Here's how the part is built. I have some questions about the finished solid (model axes, mm). A direction names the side the tool comes from. Give positions to 0.01 mm unless a question says otherwise; leave off trailing zeros. Order: outer loops, then holes, each group sorted by start corner. A loop starts at its lowest first (then second) coordinate and runs counter-clockwise, first axis right, second up. Notation, with made-up numbers: (15.25, 20) -> (55.25, 20) arc R29 ccw to (55.25, 57) -> close; hole circle Ø2 at (17.25, 64). An arc over 180 degrees is marked (long way). Write each question's results on one line, items separated by ' | '. Start each with the question number.
Q1. For faces 4 (the face through (-24, 17, -21)), 5 (the face through (1.92, 5.03, 21.45)), 6 (the face through (14.33, 16.79, -36.84)), 7 (the face through (20.49, 16.79, -36.75)), 8 (the face through (-14.328, 16.79, -6.367)), which set-ups out of +Z, -Z, +X, -X, +Y, -Y let a thin tool reach every point of the face, with its end or its side?
Q2. Thinking about a two-plate mould opening in X: for faces 1 (the face through (-19.01, 16.79, -8.22)), 2 (the face through (-13.88, 0.99, 24.24)), 3 (the face through (27.5, 1, -23)), which applies, pulls with the +X half, pulls with the -X half, needs draft (parallel to the pull), parting line crosses it, or undercut?
Q3. Imagine slicing it at B-B, the plane z = -21. Please give me the cut outline in (x, y).
Q4. I need wall thicknesses on line 1 along X through (y, z) = (27, -15); line 2 along Y through (x, z) = (13.5, -6); line 3 along Z through (x, y) = (-15.5, 13). Which ranges of each line are inside material? Lowest first, please. Write a range as [from, to].
Q5. Imagine slicing it at D-D, the plane z = 29.5. Please give me the cut outline in (x, y), then the cut area to 3 significant figures.
Q6. Imagine slicing it at C-C, the plane x = -13. Please give me the cut outline in (y, z), then the cut area to 3 significant figures.
Q7. Imagine slicing it at A-A, the plane y = 26.5. Please give me the cut outline in (x, z), then the cut area to 3 significant figures.
Q8. I'm going to push flat-ended pins straight in: pin 1 (4 mm diameter, centred on x = 1, y = 6.5, fed in from +Z); pin 2 (6.5 mm diameter, centred on y = 5.5, z = 14.5, fed in from -X); pin 3 (10 mm diameter, centred on x = -1, y = 17.5, fed in from -Z); pin 4 (4 mm diameter, centred on x = -5.5, z = -20, fed in from +Y). Where does each tip first touch, or does it pass through?
```python
from build123d import *

# Parameters (mm, degrees)
BOSS_EXTRUDE1_DEPTH = 2
BOSS_EXTRUDE2_DEPTH = 30
SKETCH3_W           = 12
SKETCH3_H           = 40
BOSS_EXTRUDE3_DEPTH = 10
CUT_EXTRUDE1_DEPTH  = 35
SKETCH6_W           = 46.796643592
SKETCH6_H           = 23.882016553
CUT_EXTRUDE2_DEPTH  = 1
FILLET1_R           = 280
FILLET2_R           = 9
FILLET3_R           = 4
FILLET4_R           = 50


with BuildPart() as part:
    # Sketch1 → Boss-Extrude1 (new body)
    with BuildSketch(Plane(origin=(0, 0, 0), x_dir=(1, 0, 0), z_dir=(0, 1, 0))):
        Polygon((-27.5, 1.096246938), (-6, -38.903753062), (6, -38.903753062), (27.5, 1.096246938), (27.5, 41.096246938), (-27.5, 41.096246938), align=None)
    extrude(amount=BOSS_EXTRUDE1_DEPTH)

    # Sketch2 → Boss-Extrude2 (add)
    with BuildSketch(Plane(origin=(0, 2, 0), x_dir=(1, 0, 0), z_dir=(0, 1, 0))):
        Polygon((-24, 9.101662984), (-24, 34.101662984), (-14.15192247, 35.838144761), (-14.499218825, 37.807760267), (-26.316911861, 35.723982135), (-26.316911861, 7.479343833), (-14.499218825, 5.395565701), (-14.15192247, 7.365181207), align=None)
        Polygon((14.15192247, 7.365181207), (14.499218825, 5.395565701), (26.316911861, 7.479343833), (26.316911861, 35.723982135), (14.499218825, 37.807760267), (14.15192247, 35.838144761), (24, 34.101662984), (24, 9.101662984), align=None)
    extrude(amount=BOSS_EXTRUDE2_DEPTH)

    # Sketch3 → Boss-Extrude3 (add)
    with BuildSketch(Plane(origin=(0, 2, 0), x_dir=(1, 0, 0), z_dir=(0, 1, 0))):
        with Locations((-0.005517933, -18.7)):
            Rectangle(SKETCH3_W, SKETCH3_H)
    extrude(amount=BOSS_EXTRUDE3_DEPTH)

    # Sketch4 → Cut-Extrude1 (cut)
    with BuildSketch(Plane.XY.offset(38.7)):
        Polygon((0, 3.110912703), (3.889087297, 7), (0, 10.889087297), (-3.889087297, 7), align=None)
    extrude(amount=-CUT_EXTRUDE1_DEPTH, mode=Mode.SUBTRACT)

    # Sketch6 → Cut-Extrude2 (cut)
    with BuildSketch(Plane(origin=(0, 2, 0), x_dir=(1, 0, 0), z_dir=(0, 1, 0))):
        with Locations((0, 21.585626422)):
            Rectangle(SKETCH6_W, SKETCH6_H)
    extrude(amount=-CUT_EXTRUDE2_DEPTH, mode=Mode.SUBTRACT)

    # Fillet1
    # the kernel refuses this fillet: 280 mm, written as the material it adds along each edge
    with BuildSketch(Plane(origin=(23.398321796, 1, -92.634586786), x_dir=(0, 1, 0), z_dir=(0, 0, 1))) as fillet1_piece_1_section:
        with BuildLine():
            CenterArc((280, 23.643180835), FILLET1_R, 180, 4.843819526)
            Line((0, 23.643180835), (0, 0))
            Line((0, 0), (1, 0))
        make_face()
    fillet1_piece_1 = extrude(amount=142.097920729, mode=Mode.PRIVATE)
    fillet1_piece_1 = split(fillet1_piece_1, bisect_by=Plane(origin=(14.446064127, 1.194161729, -5.386193094), z_dir=(-0.1736481776669284, 0, -0.9848077530122085)), keep=Keep.TOP, mode=Mode.PRIVATE)
    fillet1_piece_1 = split(fillet1_piece_1, bisect_by=Plane(origin=(14.451548954, 1.194161729, -37.816165751), z_dir=(-0.17364817766692828, 0, 0.9848077530122085)), keep=Keep.TOP, mode=Mode.PRIVATE)
    add(fillet1_piece_1)
    with BuildSketch(Plane(origin=(-23.398321796, 1, -9.644618145), x_dir=(0, 1, 0), z_dir=(0, 0, -1))) as fillet1_piece_2:
        with BuildLine():
            CenterArc((280, 23.643180835), FILLET1_R, 180, 4.843819526)
            Line((0, 23.643180835), (0, 0))
            Line((0, 0), (1, 0))
        make_face()
    extrude(amount=23.882016554)

    # Fillet2
    fillet2_edges = [part.edges().sort_by_distance(p)[0] for p in [
        (-27.5, 1, -41.096246938),
        (27.5, 1, -41.096246938),
    ]]
    fillet(fillet2_edges, radius=FILLET2_R)

    # Fillet3
    # the kernel refuses this fillet: 4 mm, written as the material it takes off along each edge
    with BuildSketch(Plane(origin=(5.994482067, 12, 48.7), x_dir=(0, -1, 0), z_dir=(0, 0, -1)), Plane(origin=(-6.005517933, 12, -11.3), x_dir=(0, -1, 0), z_dir=(0, 0, 1))) as fillet3_piece_1:
        with BuildLine():
            CenterArc((FILLET3_R, FILLET3_R), FILLET3_R, 180, 90)
            Line((0, FILLET3_R), (0, 0))
            Line((0, 0), (FILLET3_R, 0))
        make_face()
    extrude(amount=60, mode=Mode.SUBTRACT)
    with BuildSketch(Plane(origin=(15.994482067, 12, -1.3), x_dir=(0, -1, 0), z_dir=(-1, 0, 0)), Plane(origin=(-16.005517933, 12, 38.7), x_dir=(0, -1, 0), z_dir=(1, 0, 0))) as fillet3_piece_2:
        with BuildLine():
            CenterArc((FILLET3_R, FILLET3_R), FILLET3_R, 180, 90)
            Line((0, FILLET3_R), (0, 0))
            Line((0, 0), (FILLET3_R, 0))
        make_face()
    extrude(amount=32, mode=Mode.SUBTRACT)

    # Fillet4
    fillet4_edges = [part.edges().sort_by_distance(p)[0] for p in [
        (-27.5, 1, -1.096246938),
        (27.5, 1, -1.096246938),
    ]]
    fillet(fillet4_edges, radius=FILLET4_R)


solid = part.part
```
Geometry check:
1) face 4: +Y | face 5: +Z | face 6: -Z, +Y | face 7: -Z, +X, +Y | face 8: +Z, +Y
2) face 1: undercut | face 2: pulls with the -X half | face 3: pulls with the +X half
3) outline: (-27.5, 0) -> (27.5, 0) -> (27.5, 2) -> (26.32, 2) -> (26.32, 32) -> (24, 32) -> (24, 2) -> (23.4, 2) arc R280 cw to (0, 1) arc R280 cw to (-23.4, 2) -> (-24, 2) -> (-24, 32) -> (-26.32, 32) -> (-26.32, 2) -> (-27.5, 2) -> close
4) line 1: [-26.32, -24], [24, 26.32] | line 2: [0, 2] | line 3: [-37.63, -35.6], [-7.6, -5.57]
5) outline: (-11.05, 0) -> (11.05, 0) -> (11.05, 2) -> (5.99, 2) -> (5.99, 8) arc R4 ccw to (1.99, 12) -> (-2.01, 12) arc R4 ccw to (-6.01, 8) -> (-6.01, 2) -> (-11.05, 2) -> close; hole (-3.89, 7) -> (0, 3.11) -> (3.89, 7) -> (0, 10.89) -> close | area: 127 mm²
6) outline: (0, -41.1) -> (2, -41.1) -> (2, -33.53) -> (1.31, -33.53) -> (1.31, -9.64) -> (2, -9.64) -> (2, 25.88) -> (0, 25.88) -> close | area: 118 mm²
7) outline: (-26.32, -35.72) -> (-14.5, -37.81) -> (-14.15, -35.84) -> (-24, -34.1) -> (-24, -9.1) -> (-14.15, -7.37) -> (-14.5, -5.4) -> (-26.32, -7.48) -> close; (14.15, -35.84) -> (14.5, -37.81) -> (26.32, -35.72) -> (26.32, -7.48) -> (14.5, -5.4) -> (14.15, -7.37) -> (24, -9.1) -> (24, -34.1) -> close | area: 211 mm²
8) pin 1: z = 38.7 | pin 2: x = -6.01 | pin 3: through | pin 4: y = 1.11
